Autodesk Fusion 360 part; units mm, degrees
sketch "Sketch1" plane through (0, 0, 0) normal (1, 0, 0) x (0, 1, 0)
  line L0 (-20, 20) -> (20, 20) construction
  line L1 (20, 20) -> (20, -20)
  line L2 (20, -20) -> (-20, -20) construction
  line L3 (-20, -20) -> (-20, 20)
  line L4 (0, 0) -> (0, 20) construction
  line L5 (0, 0) -> (20, 0) construction
  line L6 (0, 0) -> (0, -1.6) construction
  line L7 (0, 0) -> (0, -8.6) construction
  circle A0 centre (0, -8.6) radius 6
  circle A1 centre (0, -1.6) radius 18.4 construction
  circle A2 centre (0, -1.6) radius 15.5 construction
  line L8 (0, -1.6) -> (15.5, -1.6) construction
  circle A3 centre (15.5, -1.6) radius 1.5
  circle A4 centre (7.75, 11.8234) radius 1.5
  circle A5 centre (-7.75, 11.8234) radius 1.5
  circle A6 centre (-15.5, -1.6) radius 1.5
  circle A7 centre (-7.75, -15.0234) radius 1.5
  circle A8 centre (7.75, -15.0234) radius 1.5
  line L9 (-10, 20) -> (-10, 24.8) construction
  line L10 (-10, 24.8) -> (10, 24.8)
  line L11 (10, 24.8) -> (10, 20) construction
  line L12 (-10, -20) -> (-10, -24.8) construction
  line L13 (-10, -24.8) -> (10, -24.8)
  line L14 (10, -24.8) -> (10, -20) construction
  line L15 (-11.0607, -21.0607) -> (-10, -20) construction
  line L16 (11.0607, -21.0607) -> (10, -20) construction
  line L17 (-11.0607, 21.0607) -> (-10, 20) construction
  line L18 (11.0607, 21.0607) -> (10, 20) construction
  arc A9 (-12.1213, 20) -> (-10, 22.1213) centre (-11.0607, 21.0607) ccw
  arc A10 (-10, 22.1213) -> (-12.1213, 20) centre (-11.0607, 21.0607) ccw construction
  arc A11 (10, 22.1213) -> (12.1213, 20) centre (11.0607, 21.0607) ccw
  arc A12 (12.1213, 20) -> (10, 22.1213) centre (11.0607, 21.0607) ccw construction
  arc A13 (12.1213, -20) -> (10, -22.1213) centre (11.0607, -21.0607) ccw
  arc A14 (10, -22.1213) -> (12.1213, -20) centre (11.0607, -21.0607) ccw construction
  arc A15 (-10, -22.1213) -> (-12.1213, -20) centre (-11.0607, -21.0607) ccw
  arc A16 (-12.1213, -20) -> (-10, -22.1213) centre (-11.0607, -21.0607) ccw construction
  line L19 (-10, 22.1213) -> (-10, 24.8)
  line L20 (-12.1213, 20) -> (-20, 20)
  line L21 (10, 22.1213) -> (10, 24.8)
  line L22 (12.1213, 20) -> (20, 20)
  line L23 (10, -22.1213) -> (10, -24.8)
  line L24 (12.1213, -20) -> (20, -20)
  line L25 (-10, -22.1213) -> (-10, -24.8)
  line L26 (-12.1213, -20) -> (-20, -20)
  dimension "d61" = 40
  dimension "d62" = 40
  dimension "d63" = 1.6
  dimension "d65" = 12
  dimension "d66" = 36.8
  dimension "d67" = 31
  dimension "d68" = 3
  dimension "d70" = 360
  dimension "d71" = 4.8
  dimension "d72" = 20
  dimension "d73" = 10
  dimension "d74" = 4.8
  dimension "d75" = 20
  dimension "d76" = 10
  dimension "d77" = 3
  dimension "d78" = 1.5
  dimension "d79" = 45
  dimension "d80" = 3
  dimension "d81" = 1.5
  dimension "d83" = 45
  dimension "d84" = 3
  dimension "d85" = 3
  dimension "d86" = 1.5
  dimension "d87" = 45
  dimension "d88" = 1.5
  dimension "d89" = 45
  dimension "d90" = 7
extrude "Extrude1" add sketch "Sketch1" along normal blind 4.8

Autodesk Fusion 360 part; units mm, degrees
sketch "Sketch1" plane through (0, 0, 0) normal (1, 0, 0) x (0, 1, 0)
  line L0 (-20, 20) -> (20, 20) construction
  line L1 (20, 20) -> (20, -20)
  line L2 (20, -20) -> (-20, -20) construction
  line L3 (-20, -20) -> (-20, 20)
  line L4 (0, 0) -> (20, 0) construction
  line L5 (0, 0) -> (0, 20) construction
  line L6 (-10, 20) -> (-10, 24.8) construction
  line L7 (-10, 24.8) -> (10, 24.8)
  line L8 (10, 24.8) -> (10, 20) construction
  line L9 (-10, -20) -> (-10, -24.8) construction
  line L10 (-10, -24.8) -> (10, -24.8)
  line L11 (10, -24.8) -> (10, -20) construction
  line L12 (0, 0) -> (0, -1.6) construction
  line L13 (-6, 17.0729) -> (-6, 18.5729) construction
  line L14 (-6, 18.5729) -> (6, 18.5729) construction
  line L15 (6, 18.5729) -> (6, 17.0729) construction
  line L16 (-11.0607, 21.0607) -> (-10, 20) construction
  line L17 (11.0607, 21.0607) -> (10, 20) construction
  line L18 (11.0607, -21.0607) -> (10, -20) construction
  line L19 (-11.0607, -21.0607) -> (-10, -20) construction
  arc A0 (-6, 17.0729) -> (-4.5, 18.5729) centre (-4.5, 17.0729) ccw construction
  arc A1 (-4.5, 18.5729) -> (-6, 17.0729) centre (-4.5, 17.0729) ccw
  arc A2 (4.5, 18.5729) -> (6, 17.0729) centre (4.5, 17.0729) ccw construction
  arc A3 (6, 17.0729) -> (4.5, 18.5729) centre (4.5, 17.0729) ccw
  line L20 (-6, 14.5729) -> (-6, 17.0729)
  line L21 (6, 17.0729) -> (6, 14.5729)
  arc A4 (-6, 14.5729) -> (6, 14.5729) centre (0, -1.6) ccw
  arc A5 (6, 14.5729) -> (0, 15.65) centre (0, -1.6) ccw construction
  arc A6 (0, 15.65) -> (-6, 14.5729) centre (0, -1.6) ccw construction
  line L22 (-4.5, 18.5729) -> (4.5, 18.5729)
  arc A7 (-12.1213, 20) -> (-10, 22.1213) centre (-11.0607, 21.0607) ccw
  arc A8 (-10, 22.1213) -> (-12.1213, 20) centre (-11.0607, 21.0607) ccw construction
  arc A9 (10, 22.1213) -> (12.1213, 20) centre (11.0607, 21.0607) ccw
  arc A10 (12.1213, 20) -> (10, 22.1213) centre (11.0607, 21.0607) ccw construction
  arc A11 (-10, -22.1213) -> (-12.1213, -20) centre (-11.0607, -21.0607) ccw
  arc A12 (-12.1213, -20) -> (-10, -22.1213) centre (-11.0607, -21.0607) ccw construction
  arc A13 (12.1213, -20) -> (10, -22.1213) centre (11.0607, -21.0607) ccw
  arc A14 (10, -22.1213) -> (12.1213, -20) centre (11.0607, -21.0607) ccw construction
  line L23 (-10, 22.1213) -> (-10, 24.8)
  line L24 (10, 22.1213) -> (10, 24.8)
  line L25 (12.1213, 20) -> (20, 20)
  line L26 (-12.1213, 20) -> (-20, 20)
  line L27 (-20, -20) -> (-12.1213, -20)
  line L28 (-10, -22.1213) -> (-10, -24.8)
  line L29 (10, -22.1213) -> (10, -24.8)
  line L30 (12.1213, -20) -> (20, -20)
  point P0 (0, 18.5729)
  dimension "d39" = 40
  dimension "d40" = 40
  dimension "d41" = 4.8
  dimension "d42" = 20
  dimension "d43" = 10
  dimension "d44" = 4.8
  dimension "d45" = 20
  dimension "d46" = 10
  dimension "d47" = 1.6
  dimension "d48" = 34.5
  dimension "d49" = 4
  dimension "d51" = 3
  dimension "d52" = 1.5
  dimension "d53" = 45
  dimension "d54" = 3
  dimension "d55" = 3
  dimension "d56" = 3
  dimension "d57" = 1.5
  dimension "d58" = 45
  dimension "d59" = 3
  dimension "d60" = 1.5
  dimension "d61" = 45
  dimension "d62" = 3
  dimension "d63" = 1.5
  dimension "d64" = 45
  dimension "d65" = 12
extrude "Extrude1" add sketch "Sketch1" along normal blind 4.8
Source: CAD feature listing. Evaluate the final solid. Frame: model axes, mm. A direction names the side the tool comes from. Coordinates: 2 decimals unless noted, no trailing zeros. Loops run counter-clockwise (first coordinate to the right, second up) from the corner with the lowest first, then second, coordinate; pieces in that order, holes last. Notation, with made-up numbers: M -38,-23.75 L 11,-23.75 A24 cw 11,13.25 Z; hole C 70.25,77.25 d4. An arc over 180 degrees is marked long. Put each result on its own line as item: value. Start each with the question number.
1) Pull-direction query (Z, two-part tool) for faces 4 (the face through (2, 10, -23)), 5 (the face through (2, -16, -20)), 6 (the face through (2, 0, 18.573)); classes: pulls with the +Z half, pulls with the -Z half, needs draft (parallel to the pull), parting line crosses it, or undercut.
2) Reachability of faces 1 (the face through (2, 16, -20)), 2 (the face through (2, 16, 20)), 3 (the face through (2, -6, 16)) from +Z, -Z, +X, -X, +Y, -Y: full face, straight path, thin tool, end or side. Return the list, or none.
3) Cut plane A-A on z = 16. Return the cut outline in (x, y).
4) Contact query for flat-ended pins moving along their axis: pin 1 Ø1.4 at (x, y) = (3.5, -18) entering from +Z; pin 2 Ø2.5 at (x, y) = (2, -16.5) entering from -Z; pin 3 Ø2 at (x, z) = (2.5, 23.5) entering from -Y; pin 4 Ø5 at (y, z) = (14.5, -0.5) entering from -X. Output: stop coordinate, or through.
5) Cut plane B-B on x = 3.45. Return the cut outline in (y, z), then the cut area to 3 significant figures.
6) Cut plane C-C on y = 0. Return the cut outline in (x, z), then the cut area to 4 significant figures.
7) Ray query, L1, parallel to Z at x = 4.25, y = 0; L2, parallel to Y at x = 3, z = -1.6; L3, parallel to Y at x = 1.4, z = 15. Return the intervals inside material, ascending. Write a range as from..to.
The answers:
1. face 4: needs draft
1. face 5: pulls with the -Z half
1. face 6: undercut
2. face 1: -Z, +X, -X, +Y
2. face 2: +Z, +X, -X, +Y
2. face 3: +X, -X
3. outline: M 0,-20 L 4.8,-20 L 4.8,-6 L 0,-6 Z; M 0,6 L 4.8,6 L 4.8,20 L 0,20 Z
4. pin 1: stops at z = 20
4. pin 2: stops at z = -20
4. pin 3: stops at y = -10
4. pin 4: passes through
5. outline: M -20,-20 L -12.12,-20 A1.5 cw -10,-22.12 L -10,-24.8 L 10,-24.8 L 10,-22.12 A1.5 cw 12.12,-20 L 20,-20 L 20,20 L 12.12,20 A1.5 cw 10,22.12 L 10,24.8 L -10,24.8 L -10,22.12 A1.5 cw -12.12,20 L -20,20 Z; hole M -6,14.57 A17.25 ccw long 6,14.57 L 6,17.07 A1.5 ccw 4.5,18.57 L -4.5,18.57 A1.5 ccw -6,17.07 Z
5. area: 814 mm²
6. outline: M 0,-24.8 L 4.8,-24.8 L 4.8,-18.85 L 0,-18.85 Z; M 0,18.57 L 4.8,18.57 L 4.8,24.8 L 0,24.8 Z
6. area: 58.45 mm²
7. L1: z = -24.8..-18.85, 18.57..24.8
7. L2: y = -20..-17.25, 17.25..20
7. L3: y = -20..-6, 6..20
